Model file for the job. Use its own axes, mm. Face numbers are marked on the shaded views. A direction names the side the tool comes from. Give positions to 0.01 mm unless a question says otherwise; leave off trailing zeros. Write each loop counter-clockwise with the first axis right and the second up, starting at its lowest first coordinate (ties: lowest second). Pieces come first, ordered by that corner, then holes. Notation, with made-up numbers: (-15.5, 33.5) - (1.5, 33.5) arc R7 cw to (1.5, 42.5) - close; hole circle Ø3 at (67, -8.75). An arc over 180 degrees is marked (long way). Use CSV: the item, a comma, the result in double quotes.
from build123d import *

# Parameters (mm, degrees)
BOSS_EXTRUDE1_DEPTH   = 2.5
M3_TAPPED_HOLE1_D     = 2.5
M3_TAPPED_HOLE1_DEPTH = 13.5
M3_TAPPED_HOLE1_TIP   = 0.751075774


with BuildPart() as part:
    # Sketch1 → Boss-Extrude1 (new, symmetric)
    with BuildSketch(Plane.XY):
        Polygon((40, 7.5), (0, 7.5), (0, -7.5), (5, -7.5), (5, 4.5), (40, 4.5), align=None)
    extrude(amount=BOSS_EXTRUDE1_DEPTH, both=True)

    # M3 Tapped Hole1
    with Locations(Plane.ZY):
        with Locations((0, -4), (0, 4)):
            Hole(M3_TAPPED_HOLE1_D / 2, depth=M3_TAPPED_HOLE1_DEPTH)
            with Locations((0, 0, -(M3_TAPPED_HOLE1_DEPTH + M3_TAPPED_HOLE1_TIP / 2))):  # 118° drill point
                Cone(0, M3_TAPPED_HOLE1_D / 2, M3_TAPPED_HOLE1_TIP, mode=Mode.SUBTRACT)


solid = part.part
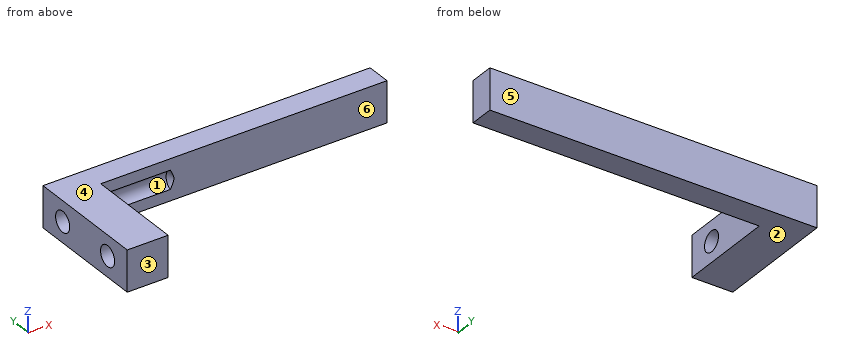
(1) Saw through at A-A, the plane y = 4. List the corners of the cut face in (x, z).
Checked values:
outline,"(0, -2.5) - (5, -2.5) - (5, -1.25) - (0, -1.25) - close; (0, 1.25) - (5, 1.25) - (5, 2.5) - (0, 2.5) - close"
(2) Saw through at C-C, the plane z = 0.6. Count the separate pieces of the cut face and the enclosed holes in it, then the cut area to 3 significant figures.
Checked values:
separate pieces,"3"
enclosed holes,"0"
area,"153 mm^2"
(3) Flat gauge pins, fed straight in: P1, Ø3, axis at y = -2, z = -1, coming from the +X side; P2, Ø2, axis at x = 33, z = 1.5, coming from the -Y side. Where does each tip first touch, or does it go through?
Checked values:
P1,"stops at x = 5"
P2,"stops at y = 4.5"
(4) Pull direction Z, two halves, no side cores. Call the marked faces 1, 2, 3 and 4: released by +Z, released by -Z, zero draft, split by the parting line, or undercut.
Checked values:
face 1,"undercut"
face 2,"released by -Z"
face 3,"zero draft"
face 4,"released by +Z"
(5) Saw through at B-B, the plane x = 10. List the corners of the cut face in (y, z), then the cut area to 3 significant figures.
Checked values:
outline,"(4.5, -2.5) - (7.5, -2.5) - (7.5, 2.5) - (4.5, 2.5) - (4.5, 1.15) arc R1.25 cw to (4.5, -1.15) - close"
area,"13.8 mm^2"
(6) Saw through at D-D, the plane y = 0.25. List the corners of the cut face in (x, z).
Checked values:
outline,"(0, -2.5) - (5, -2.5) - (5, 2.5) - (0, 2.5) - close"
(7) Wall check: probe 1 along Z at (x, y) = (4.25, 4); probe 2 along Y at (x, z) = (1.6, 0); probe 3 along X at (y, z) = (-0.5, -2). Give the ranges that are in metal, low to high. Write a range as [from, to].
Checked values:
probe 1,"z = [-2.5, -1.25], [1.25, 2.5]"
probe 2,"y = [-7.5, -5.25], [-2.75, 2.75], [5.25, 7.5]"
probe 3,"x = [0, 5]"
(8) 3-axis set-ups, long thin cutter, end or side, ignore diameter. For the marked faces 5 and 6: which of +Z, -Z, +X, -X, +Y, -Y reach the whole face in a straight line?
Checked values:
face 5,"+Z, -Z, +X, -X, +Y"
face 6,"+Z, -Z, +X, -Y"
